```python
from build123d import *

# Parameters (mm, degrees)
BOSS_EXTRUDE1_DEPTH = 15.24
SKETCH2_3_R         = 2.38125
BOSS_EXTRUDE2_DEPTH = 1.5875


with BuildPart() as part:
    # Sketch2 → Boss-Extrude1 (new body)
    with BuildSketch(Plane(origin=(0, 0, 0), x_dir=(1, 0, 0), z_dir=(0, 1, 0))):
        Polygon((-12.7, 12.7), (2.553439785, 12.7), (1.895875755, 14.2875), (-14.2875, 14.2875), (-14.2875, -4.719098556), (-12.7, -8.551662587), align=None)
        Polygon((1.895875755, 14.2875), (2.553439785, 12.7), (4.271737403, 12.7), (3.614173373, 14.2875), align=None)
        Polygon((3.614173373, 14.2875), (4.271737403, 12.7), (12.7, 12.7), (12.7, 4.271737403), (14.2875, 3.614173373), (14.2875, 14.2875), align=None)
        Polygon((14.2875, 1.895875755), (12.7, 2.553439785), (12.7, -12.7), (-8.551662587, -12.7), (-4.719098556, -14.2875), (14.2875, -14.2875), align=None)
        Polygon((12.7, 4.271737403), (12.7, 2.553439785), (14.2875, 1.895875755), (14.2875, 3.614173373), align=None)
        Polygon((-12.7, -12.7), (-12.7, -8.551662587), (-14.2875, -4.719098556), (-14.2875, -8.86743597), align=None)
        Polygon((-8.86743597, -14.2875), (-12.7, -12.7), (-14.2875, -8.86743597), (-14.2875, -14.2875), align=None)
        Polygon((-8.551662587, -12.7), (-12.7, -12.7), (-8.86743597, -14.2875), (-4.719098556, -14.2875), align=None)
    extrude(amount=BOSS_EXTRUDE1_DEPTH)

    # Sketch2_3 → Boss-Extrude2 (add)
    # profile 1 of 2: a face of its own
    with BuildSketch(Plane(origin=(0, 0, 0), x_dir=(1, 0, 0), z_dir=(0, 1, 0))):
        Polygon((-14.2875, 14.2875), (3.614173373, 14.2875), (-6.243738443, 38.086604402), (-29.710278569, 28.36644522), (-14.2875, -8.86743597), align=None)
        with Locations(Location((-20.225507313, 22.061531474, 0), (0, 0, 270))):
            Circle(SKETCH2_3_R, mode=Mode.SUBTRACT)
        with Locations(Location((-8.492237251, 26.921611065, 0), (0, 0, 270))):
            Circle(SKETCH2_3_R, mode=Mode.SUBTRACT)
    # profile 2 of 2: a face of its own
    with BuildSketch(Plane(origin=(0, 0, 0), x_dir=(1, 0, 0), z_dir=(0, 1, 0))):
        Polygon((14.2875, 3.614173373), (14.2875, -14.2875), (-8.86743597, -14.2875), (28.36644522, -29.710278569), (38.086604402, -6.243738443), align=None)
        with Locations(Location((26.921611065, -8.492237251, 0), (0, 0, 270))):
            Circle(SKETCH2_3_R, mode=Mode.SUBTRACT)
        with Locations(Location((22.061531474, -20.225507313, 0), (0, 0, 270))):
            Circle(SKETCH2_3_R, mode=Mode.SUBTRACT)
    extrude(amount=BOSS_EXTRUDE2_DEPTH)


solid = part.part
```
CAD build for the part. Positions are in the model's coordinates, mm. A direction names the side the tool comes from. Give positions to 0.01 mm unless a question says otherwise; leave off trailing zeros. Order: outer loops, then holes, each group sorted by start corner. A loop starts at its lowest first (then second) coordinate and runs counter-clockwise, first axis right, second up. Notation, with made-up numbers: M 34,60 L 92,60 A26 ccw 92,83 Z; hole C -20.75,50.5 d11. An arc over 180 degrees is marked long. Put each result on its own line as item: value. Start each with the question number.
(1) Saw through at C-C, the plane x = -1. Write the cut outline in (y, z).
(2) Saw through at A-A, the plane z = -5.5. Write the cut outline in (x, y).
(3) Flat gauge pins, fed straight in: pin 1 Ø5 at (x, z) = (5.5, 19) entering from +Y; pin 2 Ø4.5 at (y, z) = (8.5, 0.5) entering from +X; pin 3 Ø7.5 at (x, y) = (4.5, 9.5) entering from +Z. Where does each tip first touch, or does it go through?
(4) Drill centre lines: line 1 along Z through (x, y) = (-8.5, 13.75); line 2 along Y through (x, z) = (-11, -25.5). Where is each one in solid material? Low to high.
(5) Saw through at B-B, the plane y = 7.5. Write the cut outline in (x, z), then the cut area to 3 significant figures.
(6) Saw through at D-D, the plane z = -22. Write the cut outline in (x, y), then the cut area to 3 significant figures.
(7) Which spindle directions (+Z, -Z, +X, -X, +Y, -Y) get a long thin tool onto all of the face, cutting with end or side? Do faces 1 (the flat face through (-1.246, 0.783, -26.02)), 2 (the flat face through (0, 8, 12.7)). Say none if no direction does.
(8) Mould opens along X. For faces 3 (the flat face through (14.288, 8, 0)), 4 (the flat face through (0, 8, -12.7)), 5 (the flat face through (-14.288, 8, 0)), 6 (the flat face through (-4, 0, -14)) say: +X half, -X half, draft (parallel to the pull), parting line (faces both ways), or undercut.
Check result:
1. outline: M 0,-25.43 L 1.59,-25.43 L 1.59,-14.29 L 15.24,-14.29 L 15.24,-12.7 L 0,-12.7 Z; M 0,12.7 L 15.24,12.7 L 15.24,14.29 L 1.59,14.29 L 1.59,17.55 L 0,17.55 Z
2. outline: M -20.24,0 L -12.7,0 L -12.7,15.24 L -14.29,15.24 L -14.29,1.59 L -20.24,1.59 Z; M 12.7,0 L 14.29,0 L 14.29,15.24 L 12.7,15.24 Z
3. pin 1: stops at y = 1.59
3. pin 2: stops at x = 14.29
3. pin 3: stops at z = 14.29
4. line 1: z = -14.29 to -12.7, 12.7 to 14.29
4. line 2: y = 0 to 1.59
5. outline: M -14.29,-14.29 L 14.29,-14.29 L 14.29,14.29 L -14.29,14.29 Z; hole M -12.7,-12.7 L 12.7,-12.7 L 12.7,12.7 L -12.7,12.7 Z
5. area: 171 mm2
6. outline: M -27.07,0 L -22.61,0 L -22.61,1.59 L -27.07,1.59 Z; M -17.85,0 L 0.42,0 L 0.42,1.59 L -17.85,1.59 Z
6. area: 36.1 mm2
7. face 1: -Z, +X, +Y, -Y
7. face 2: +Y, -Y
8. face 3: +X half
8. face 4: undercut
8. face 5: -X half
8. face 6: draft
